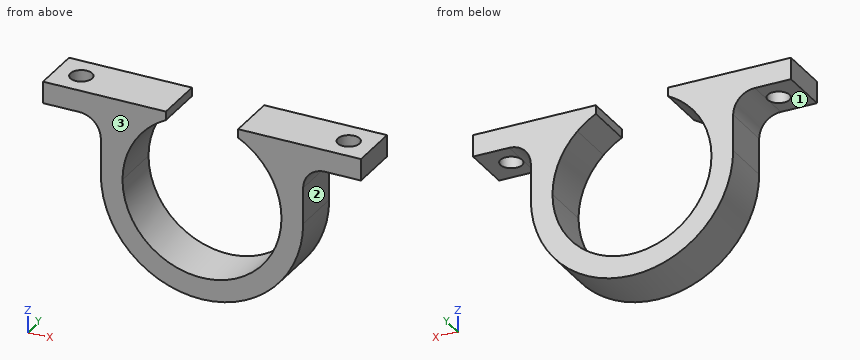
from build123d import *

# Parameters (mm, degrees)
SKETCH1_W           = 8
SKETCH1_H           = 3
BOSS_EXTRUDE2_DEPTH = 7
FILLET3_R           = 3
FILLET4_R           = 3
SKETCH3_R           = 1.5
CUT_EXTRUDE1_DEPTH  = 7


with BuildPart() as part:
    # Sketch1 → Boss-Extrude2 (new body)
    with BuildSketch(Plane(origin=(0, 0, 0), x_dir=(1, 0, 0), z_dir=(0, 1, 0))):
        with Locations((-18, -9.5)):
            Rectangle(SKETCH1_W, SKETCH1_H)
        with BuildLine():
            Line((-14, -8), (-11.489125293, -8))
            ThreePointArc((-11.489125293, -8), (-13.357540082, -4.192388692), (-14, 0))
            Line((-14, 0), (-14, -8))
        make_face()
        with BuildLine():
            Line((-14, -11), (-8.660254038, -11))
            ThreePointArc((-8.660254038, -11), (-10.185743559, -9.604719056), (-11.489125293, -8))
            Line((-11.489125293, -8), (-14, -8))
            Line((-14, -8), (-14, -11))
        make_face()
        with BuildLine():
            ThreePointArc((-11.489125293, -8), (-10.185743559, -9.604719056), (-8.660254038, -11))
            Line((-8.660254038, -11), (-5, -11))
            Line((-5, -11), (-5, -9.797958971))
            ThreePointArc((-5, -9.797958971), (-6.338986528, -8.989841478), (-7.549834435, -8))
            Line((-7.549834435, -8), (-11.489125293, -8))
        make_face()
        with BuildLine():
            ThreePointArc((-14, 0), (-13.357540082, -4.192388692), (-11.489125293, -8))
            Line((-11.489125293, -8), (-7.549834435, -8))
            ThreePointArc((-7.549834435, -8), (-10.100697471, -4.356134824), (-11, 0))
            Line((-11, 0), (-14, 0))
        make_face()
        with BuildLine():
            Line((11, 0), (14, 0))
            ThreePointArc((14, 0), (0, 14), (-14, 0))
            Line((-14, 0), (-11, 0))
            ThreePointArc((-11, 0), (0, 11), (11, 0))
        make_face()
        with BuildLine():
            Line((7.549834435, -8), (11.489125293, -8))
            ThreePointArc((11.489125293, -8), (13.357540082, -4.192388692), (14, 0))
            Line((14, 0), (11, 0))
            ThreePointArc((11, 0), (10.100697471, -4.356134824), (7.549834435, -8))
        make_face()
        with BuildLine():
            Line((5, -11), (8.660254038, -11))
            ThreePointArc((8.660254038, -11), (10.185743559, -9.604719056), (11.489125293, -8))
            Line((11.489125293, -8), (7.549834435, -8))
            ThreePointArc((7.549834435, -8), (6.338986528, -8.989841478), (5, -9.797958971))
            Line((5, -9.797958971), (5, -11))
        make_face()
        with BuildLine():
            Line((11.489125293, -8), (14, -8))
            Line((14, -8), (14, 0))
            ThreePointArc((14, 0), (13.357540082, -4.192388692), (11.489125293, -8))
        make_face()
        with BuildLine():
            Line((8.660254038, -11), (14, -11))
            Line((14, -11), (14, -8))
            Line((14, -8), (11.489125293, -8))
            ThreePointArc((11.489125293, -8), (10.185743559, -9.604719056), (8.660254038, -11))
        make_face()
        with Locations((18, -9.5)):
            Rectangle(SKETCH1_W, SKETCH1_H)
    extrude(amount=BOSS_EXTRUDE2_DEPTH)

    # Fillet3
    fillet3_edges = [part.edges().sort_by_distance(p)[0] for p in [
        (14, 3.5, 8),
    ]]
    fillet(fillet3_edges, radius=FILLET3_R)

    # Fillet4
    fillet4_edges = [part.edges().sort_by_distance(p)[0] for p in [
        (-14, 3.5, 8),
    ]]
    fillet(fillet4_edges, radius=FILLET4_R)

    # Sketch3 → Cut-Extrude1 (cut)
    with BuildSketch(Plane.XY.offset(11)):
        with Locations((-18.5, 3.5)):
            Circle(SKETCH3_R)
        with Locations((18.5, 3.5)):
            Circle(SKETCH3_R)
    extrude(amount=-CUT_EXTRUDE1_DEPTH, mode=Mode.SUBTRACT)


solid = part.part
For this review, take the finished solid that the model builds, in its own axes (mm). Face numbers are marked on the shaded views. A direction names the side the tool comes from. Round coordinates to 2 decimals unless told otherwise and drop trailing zeros. Write each loop counter-clockwise with the first axis right and the second up, starting at its lowest first coordinate (ties: lowest second). Pieces come first, ordered by that corner, then holes. Notation, with made-up numbers: (82, 30) -> (100, 30) arc R24 cw to (100, 58) -> close; hole circle Ø4 at (80.25, 10). An arc over 180 degrees is marked (long way). Use CSV: the item, a comma, the result in double quotes.
(1) Consider section B-B, the plane z = -1.25. Give the boundary of the cut face in (x, y), plus the area to 3 significant figures.
Computed values:
outline,"(-13.94, 0) -> (-10.93, 0) -> (-10.93, 7) -> (-13.94, 7) -> close; (10.93, 0) -> (13.94, 0) -> (13.94, 7) -> (10.93, 7) -> close"
area,"42.2 mm²"
(2) To check wall thickness, follow L1, parallel to Y at x = -18.5, z = 9.6; L2, parallel to X at y = 4.25, z = -4.75; L3, parallel to X at y = 5, z = 7. State the ranges of each line that lie inside material, in increasing order. Write a range as [from, to].
Computed values:
L1,"[0, 2], [5, 7]"
L2,"[-13.17, -9.92], [9.92, 13.17]"
L3,"[-14.76, -8.49], [8.49, 14.76]"
(3) For the marked faces 1, 2 and 3, list the 3-axis set-ups (+Z, -Z, +X, -X, +Y, -Y) from which the entire face can be reached by the end or side of a thin tool; tool diameter is ignored.
Computed values:
face 1,"-Z, -X, +Y, -Y"
face 2,"-Z, +X, +Y, -Y"
face 3,"+Z, -Z, +X, -X, -Y"
(4) Clearance check with flat-ended pins moving along their axes: P1, Ø3, axis at y = 1, z = 1.5, coming from the -X side; P2, Ø3, axis at y = 2, z = 1, coming from the +X side; P3, Ø1.5, axis at y = 4.5, z = -2, coming from the -X side; P4, Ø2.5, axis at x = 18.5, y = 3.5, coming from the +Z side. State where each tip first meets the part, or that it passes through.
Computed values:
P1,"x = -14"
P2,"x = 14"
P3,"x = -13.94"
P4,"through"
(5) Consider section A-A, the plane x = -18.5. Give the boundary of the cut face in (y, z), plus the area to 3 significant figures.
Computed values:
outline,"(0, 8) -> (2, 8) -> (2, 11) -> (0, 11) -> close; (5, 8) -> (7, 8) -> (7, 11) -> (5, 11) -> close"
area,"12.0 mm²"
(6) Consider section D-D, the plane x = 0. Give the boundary of the cut face in (y, z), plus the area to 3 significant figures.
Computed values:
outline,"(0, -14) -> (7, -14) -> (7, -11) -> (0, -11) -> close"
area,"21.0 mm²"
(7) Consider section C-C, the plane y = 6. Give the boundary of the cut face in (x, z).
Computed values:
outline,"(-22, 8) -> (-17, 8) arc R3 cw to (-14, 5) -> (-14, 0) arc R14 ccw to (14, 0) -> (14, 5) arc R3 cw to (17, 8) -> (22, 8) -> (22, 11) -> (5, 11) -> (5, 9.8) arc R11 cw (long way) to (-5, 9.8) -> (-5, 11) -> (-22, 11) -> close"
